```python
from build123d import *

# Parameters (mm, degrees)
F3_D     = 6.6
F5_DEPTH = 25


# Not quite as in the source:
# - a feature names something its author has since deleted; it is built from what else it names


with BuildPart() as f1:
    # F0 (on Right) → F1 (revolve)
    with BuildSketch(Plane.YZ):
        Polygon((-11.5, 40), (-40, 40), (-40, 38), (-58, 38), (-58, 30), (-40, 30), (-40, 0), (-30, 0), (-30, 28), (-11.5, 28), align=None)
    revolve(axis=Axis((0, 0, 32.5555), (0, 0, 1)))

    # F3 (through all)
    with Locations(Plane.XY.offset(40)):
        with Locations((-50, 0), (0, 50), (50, 0), (0, -50)):
            Hole(F3_D / 2)

    # F4 (on face) → F5 (cut)
    with BuildSketch(Plane.XY.offset(38)):
        with BuildLine():
            Line((-40, -42), (-40, 0))
            Line((-40, 0), (-46.7, 0))
            ThreePointArc((-46.7, 0), (-50, -3.3), (-53.3, 0))
            Line((-53.3, 0), (-58, 0))
            ThreePointArc((-58, 0), (-53.310411741, -22.8473193176), (-40, -42))
        make_face()
        with BuildLine():
            Line((-46.7, 0), (-40, 0))
            Line((-40, 0), (-40, 42))
            ThreePointArc((-40, 42), (-53.310411741, 22.8473193176), (-58, 0))
            Line((-58, 0), (-53.3, 0))
            ThreePointArc((-53.3, 0), (-50, 3.3), (-46.7, 0))
        make_face()
        with BuildLine():
            Line((-40, -44.474773109), (-40, -42))
            ThreePointArc((-40, -42), (-53.310411741, -22.8473193176), (-58, 0))
            Line((-58, 0), (-66.5342658758, 0))
            Line((-66.5342658758, 0), (-66.5342658758, -44.474773109))
            Line((-66.5342658758, -44.474773109), (-40, -44.474773109))
        make_face()
        with BuildLine():
            ThreePointArc((-58, 0), (-53.310411741, 22.8473193176), (-40, 42))
            Line((-40, 42), (-40, 51.5907406807))
            Line((-40, 51.5907406807), (-66.5342658758, 51.5907406807))
            Line((-66.5342658758, 51.5907406807), (-66.5342658758, 0))
            Line((-66.5342658758, 0), (-58, 0))
        make_face()
    extrude(amount=-F5_DEPTH, mode=Mode.SUBTRACT)


solid = f1.part
```
The listing builds one solid part. Answer for the finished solid, in the listing's coordinates (mm). A direction names the side the tool comes from. Round coordinates to 2 decimals unless told otherwise and drop trailing zeros. Write each loop counter-clockwise with the first axis right and the second up, starting at its lowest first coordinate (ties: lowest second). Pieces come first, ordered by that corner, then holes. Notation, with made-up numbers: (-31, 12.25) -> (2, 12.25) arc R23 cw to (2, 36.25) -> close; hole circle Ø11 at (89, -9). An arc over 180 degrees is marked (long way). Write item = value, one per line.
1) Section C-C on y = -50 is taken. Write down the section's boundary in (x, z), plus the area to 3 significant figures.
Check values:
outline = (-29.39, 30) -> (-3.3, 30) -> (-3.3, 38) -> (-29.39, 38) -> close; (3.3, 30) -> (29.39, 30) -> (29.39, 38) -> (3.3, 38) -> close
area = 418 mm²
2) Section B-B on x = 49 is taken. Write down the section's boundary in (y, z).
Check values:
outline = (-31.03, 30) -> (-3.14, 30) -> (-3.14, 38) -> (-31.03, 38) -> close; (3.14, 30) -> (31.03, 30) -> (31.03, 38) -> (3.14, 38) -> close
3) Which of the six approach directions +Z, -Z, +X, -X, +Y, -Y give full straight-line access (tool end or side, diameter ignored) to faces 1 (the cylindrical face through (1.32, 29.97, 14.2)), 2 (the flat face through (30, -6, 0)), 3 (the flat face through (42, -1, 38))?
Check values:
face_1 = -Z
face_2 = -Z, +X, -X, +Y, -Y
face_3 = +Z
4) Given pin 1 (8 mm diameter, centred on x = 30, z = 24.5, fed in from +Y); pin 2 (2 mm diameter, centred on x = -16.5, y = -23.5, fed in from -Z); pin 3 (6 mm diameter, centred on x = 38.5, z = 35.5, fed in from +Y), each flat-ended and moving along its own axis, determine where each tip first touches the part or whether it passes through.
Check values:
pin_1 = 30.4
pin_2 = 28
pin_3 = 45.87
5) Section A-A on x = 0 is taken. Write down the section's boundary in (y, z), plus the area to 3 significant figures.
Check values:
outline = (-58, 30) -> (-53.3, 30) -> (-53.3, 38) -> (-58, 38) -> close; (-46.7, 30) -> (-40, 30) -> (-40, 0) -> (-30, 0) -> (-30, 28) -> (-11.5, 28) -> (-11.5, 40) -> (-40, 40) -> (-40, 38) -> (-46.7, 38) -> close; (11.5, 28) -> (30, 28) -> (30, 0) -> (40, 0) -> (40, 30) -> (46.7, 30) -> (46.7, 38) -> (40, 38) -> (40, 40) -> (11.5, 40) -> close; (53.3, 30) -> (58, 30) -> (58, 38) -> (53.3, 38) -> close
area = 1,430 mm²
6) Section D-D on z = 7 is taken. Write down the section's boundary in (x, y).
Check values:
outline = circle Ø80 at (0, 0); hole circle Ø60 at (0, 0)
7) Straight lines are drawn through the part: line 1 along Z through (x, y) = (46, 10); line 2 along Z through (x, y) = (27, 5.5); line 3 along Y through (x, z) = (50, 35.75). For each, find the intervals that lie inside material, in ascending order. Write a range as [from, to].
Check values:
line_1 = [30, 38]
line_2 = [28, 40]
line_3 = [-29.39, -3.3], [3.3, 29.39]
